Could you check a few things on this model? Use its own coordinates, in mm. Face numbers are marked on the shaded views. A direction names the side the tool comes from. Give positions to 0.01 mm unless a question says otherwise; leave off trailing zeros.
1. For the marked faces 1, 2 and 3, which set-ups out of +Z, -Z, +X, -X, +Y, -Y let a thin tool reach every point of the face, with its end or its side?
2. I need wall thicknesses on line 1 along X through (y, z) = (43, -130); line 2 along Y through (x, z) = (172, 88); line 3 along X through (y, z) = (-480, 148.5). Which ranges of each line are inside material? Lowest first, please.
3. Imagine slicing it at B-B (y = -230). Count the separate pieces of the cut face and the enclosed holes in it, plus the area to 3 significant figures.
4. Thinking about a two-plate mould opening in Y: for the marked faces 4, 5, 6 and 7, which applies, +Y half, -Y half, draft (parallel to the pull), parting line (faces both ways), or undercut?
5. For P1, Ø1.5, axis at x = 112.5, y = -453.5, coming from the +Z side; P2, Ø4, axis at x = 325, z = -55, coming from the +Y side; P3, Ø12, axis at y = -140, z = 74.5, coming from the +X side, each with a flat end and sliding along its axis, tell me the tip position at first contact or that it passes through.
```python
from build123d import *

# Parameters (mm, degrees)
SKETCH2_R           = 30
SKETCH2_R_2         = 105
SKETCH2_R_3         = 28.090856429
SKETCH2_R_4         = 15
BOSS_EXTRUDE2_DEPTH = 50
SKETCH5_R           = 30
CUT_EXTRUDE1_DEPTH  = 10
CHAMFER2_SIZE       = 10
BOSS_EXTRUDE3_START = 100
SKETCH6_R           = 145
SKETCH6_R_2         = 105
BOSS_EXTRUDE3_DEPTH = 100
CUT_EXTRUDE2_START  = -10
SKETCH9_R           = 30
SKETCH9_R_2         = 15
CUT_EXTRUDE2_DEPTH  = 10
SWEEP3_OUTLINE_R    = 145
SWEEP3_OUTLINE_R_2  = 105
SWEEP3_ANGLE        = 90
SKETCH12_R          = 145
SKETCH12_R_2        = 105
BOSS_EXTRUDE5_DEPTH = 100
BOSS_EXTRUDE6_DEPTH = 50
SKETCH14_R          = 105
CUT_EXTRUDE5_DEPTH  = 50
SKETCH17_R          = 30
SKETCH17_R_2        = 15
CUT_EXTRUDE6_DEPTH  = 10
SKETCH18_R          = 15
CUT_EXTRUDE7_DEPTH  = 100
CHAMFER3_SIZE       = 10


# Read off the part's stored shape, not the designer's step: Sweep3
with BuildPart() as part:
    # Sketch2 → Boss-Extrude2 (new body)
    # profile 1 of 5: a face of its own
    with BuildSketch(Plane(origin=(0, 0, 0), x_dir=(1, 0, 0), z_dir=(0, 1, 0))):
        with BuildLine():
            Line((-180, -130), (-180, -160))
            ThreePointArc((-180, -160), (-174.142135624, -174.142135624), (-160, -180))
            Line((-160, -180), (160, -180))
            ThreePointArc((160, -180), (174.142135624, -174.142135624), (180, -160))
            Line((180, -160), (180, 160))
            ThreePointArc((180, 160), (174.142135624, 174.142135624), (160, 180))
            Line((160, 180), (-160, 180))
            ThreePointArc((-160, 180), (-174.142135624, 174.142135624), (-180, 160))
            Line((-180, 160), (-180, -130))
        make_face()
        with Locations((-130, -130)):
            Circle(SKETCH2_R, mode=Mode.SUBTRACT)
        with Locations((130, -130)):
            Circle(SKETCH2_R, mode=Mode.SUBTRACT)
        with Locations((-130, 130)):
            Circle(SKETCH2_R, mode=Mode.SUBTRACT)
        with Locations(Location((0, 0, 0), (0, 0, 270))):
            Circle(SKETCH2_R_2, mode=Mode.SUBTRACT)
        with Locations((130, 130)):
            Circle(SKETCH2_R_3, mode=Mode.SUBTRACT)
    # profile 2 of 5: a face of its own
    with BuildSketch(Plane(origin=(0, 0, 0), x_dir=(1, 0, 0), z_dir=(0, 1, 0))):
        with Locations((-130, 130)):
            Circle(SKETCH2_R)
        with Locations(Location((-130, 130, 0), (0, 0, 270))):
            Circle(SKETCH2_R_4, mode=Mode.SUBTRACT)
    # profile 3 of 5: a face of its own
    with BuildSketch(Plane(origin=(0, 0, 0), x_dir=(1, 0, 0), z_dir=(0, 1, 0))):
        with Locations((130, 130)):
            Circle(SKETCH2_R_3)
        with Locations(Location((130, 130, 0), (0, 0, 270))):
            Circle(SKETCH2_R_4, mode=Mode.SUBTRACT)
    # profile 4 of 5: a face of its own
    with BuildSketch(Plane(origin=(0, 0, 0), x_dir=(1, 0, 0), z_dir=(0, 1, 0))):
        with Locations((-130, -130)):
            Circle(SKETCH2_R)
        with Locations(Location((-130, -130, 0), (0, 0, 270))):
            Circle(SKETCH2_R_4, mode=Mode.SUBTRACT)
    # profile 5 of 5: a face of its own
    with BuildSketch(Plane(origin=(0, 0, 0), x_dir=(1, 0, 0), z_dir=(0, 1, 0))):
        with Locations((130, -130)):
            Circle(SKETCH2_R)
        with Locations(Location((130, -130, 0), (0, 0, 270))):
            Circle(SKETCH2_R_4, mode=Mode.SUBTRACT)
    extrude(amount=BOSS_EXTRUDE2_DEPTH)

    # Sketch5 → Cut-Extrude1 (cut)
    with BuildSketch(Plane(origin=(0, 50, 0), x_dir=(1, 0, 0), z_dir=(0, 1, 0))):
        with Locations(Location((-130, 130, 0), (0, 0, 270))):
            Circle(SKETCH5_R)
        with Locations(Location((130, 130, 0), (0, 0, 270))):
            Circle(SKETCH5_R)
        with Locations(Location((-130, -130, 0), (0, 0, 270))):
            Circle(SKETCH5_R)
    extrude(amount=-CUT_EXTRUDE1_DEPTH, mode=Mode.SUBTRACT)

    # Chamfer2
    chamfer2_edges = [part.edges().sort_by_distance(p)[0] for p in [
        (0, 50, -105),
    ]]
    chamfer(chamfer2_edges, length=CHAMFER2_SIZE)

    # Sketch6 → Boss-Extrude3 (add)
    with BuildSketch(Plane.XZ.offset(BOSS_EXTRUDE3_START)):
        with Locations(Location((0, 0, 0), (0, 0, 90))):
            Circle(SKETCH6_R)
        with Locations(Location((0, 0, 0), (0, 0, 270))):
            Circle(SKETCH6_R_2, mode=Mode.SUBTRACT)
    extrude(amount=-BOSS_EXTRUDE3_DEPTH)

    # Sketch9 → Cut-Extrude2 (cut)
    with BuildSketch(Plane(origin=(0, 50, 0), x_dir=(1, 0, 0), z_dir=(0, 1, 0)).offset(CUT_EXTRUDE2_START)):
        with Locations(Location((130, -130, 0), (0, 0, 270))):
            Circle(SKETCH9_R)
        with Locations(Location((130, -130, 0), (0, 0, 270))):
            Circle(SKETCH9_R_2, mode=Mode.SUBTRACT)
    extrude(amount=CUT_EXTRUDE2_DEPTH, mode=Mode.SUBTRACT)

    # Sweep3 outline → Sweep3 (revolve)
    with BuildSketch(Plane(origin=(260, -100, 0), x_dir=(-1, 0, 0), z_dir=(0, 1, 0))):
        with Locations((260, 0)):
            Circle(SWEEP3_OUTLINE_R)
        with Locations((260, 0)):
            Circle(SWEEP3_OUTLINE_R_2, mode=Mode.SUBTRACT)
    revolve(axis=Axis((260, -100, 0), (0, 0, 1)), revolution_arc=SWEEP3_ANGLE)

    # Sketch12 → Boss-Extrude5 (add)
    with BuildSketch(Plane(origin=(260, 0, 0), x_dir=(0, 0, -1), z_dir=(1, 0, 0))):
        with Locations(Location((0, -360, 0), (0, 0, 270))):
            Circle(SKETCH12_R)
        with Locations(Location((0, -360, 0), (0, 0, 270))):
            Circle(SKETCH12_R_2, mode=Mode.SUBTRACT)
    extrude(amount=BOSS_EXTRUDE5_DEPTH)

    # Sketch13 → Boss-Extrude6 (add)
    with BuildSketch(Plane(origin=(360, 0, 0), x_dir=(0, 0, -1), z_dir=(1, 0, 0))):
        with BuildLine():
            Line((-170, -540), (170, -540))
            ThreePointArc((170, -540), (177.071067812, -537.071067812), (180, -530))
            Line((180, -530), (180, -190))
            ThreePointArc((180, -190), (177.071067812, -182.928932188), (170, -180))
            Line((170, -180), (-170, -180))
            ThreePointArc((-170, -180), (-177.071067812, -182.928932188), (-180, -190))
            Line((-180, -190), (-180, -530))
            ThreePointArc((-180, -530), (-177.071067812, -537.071067812), (-170, -540))
        make_face()
    extrude(amount=BOSS_EXTRUDE6_DEPTH)

    # Sketch14 → Cut-Extrude5 (cut)
    with BuildSketch(Plane(origin=(410, 0, 0), x_dir=(0, 0, -1), z_dir=(1, 0, 0))):
        with Locations(Location((0, -369.029004143, 0), (0, 0, 90))):
            Circle(SKETCH14_R)
    extrude(amount=-CUT_EXTRUDE5_DEPTH, mode=Mode.SUBTRACT)

    # Sketch17 → Cut-Extrude6 (cut)
    # profile 1 of 4: a face of its own
    with BuildSketch(Plane(origin=(410, 0, 0), x_dir=(0, 0, -1), z_dir=(1, 0, 0))):
        with Locations(Location((-130, -230, 0), (0, 0, 90))):
            Circle(SKETCH17_R)
        with Locations(Location((-130, -230, 0), (0, 0, 90))):
            Circle(SKETCH17_R_2, mode=Mode.SUBTRACT)
    # profile 2 of 4: a face of its own
    with BuildSketch(Plane(origin=(410, 0, 0), x_dir=(0, 0, -1), z_dir=(1, 0, 0))):
        with Locations(Location((-130, -490, 0), (0, 0, 90))):
            Circle(SKETCH17_R)
        with Locations(Location((-130, -490, 0), (0, 0, 90))):
            Circle(SKETCH17_R_2, mode=Mode.SUBTRACT)
    # profile 3 of 4: a face of its own
    with BuildSketch(Plane(origin=(410, 0, 0), x_dir=(0, 0, -1), z_dir=(1, 0, 0))):
        with Locations(Location((130, -490, 0), (0, 0, 90))):
            Circle(SKETCH17_R)
        with Locations(Location((130, -490, 0), (0, 0, 90))):
            Circle(SKETCH17_R_2, mode=Mode.SUBTRACT)
    # profile 4 of 4: a face of its own
    with BuildSketch(Plane(origin=(410, 0, 0), x_dir=(0, 0, -1), z_dir=(1, 0, 0))):
        with Locations(Location((130, -230, 0), (0, 0, 90))):
            Circle(SKETCH17_R)
        with Locations(Location((130, -230, 0), (0, 0, 90))):
            Circle(SKETCH17_R_2, mode=Mode.SUBTRACT)
    extrude(amount=-CUT_EXTRUDE6_DEPTH, mode=Mode.SUBTRACT)

    # Sketch18 → Cut-Extrude7 (cut)
    with BuildSketch(Plane(origin=(410, 0, 0), x_dir=(0, 0, -1), z_dir=(1, 0, 0))):
        with Locations(Location((-130, -230, 0), (0, 0, 90))):
            Circle(SKETCH18_R)
        with Locations(Location((130, -230, 0), (0, 0, 90))):
            Circle(SKETCH18_R)
        with Locations(Location((-130, -490, 0), (0, 0, 90))):
            Circle(SKETCH18_R)
        with Locations(Location((130, -490, 0), (0, 0, 90))):
            Circle(SKETCH18_R)
    extrude(amount=-CUT_EXTRUDE7_DEPTH, mode=Mode.SUBTRACT)

    # Chamfer3
    chamfer3_edges = [part.edges().sort_by_distance(p)[0] for p in [
        (410, -474.029004143, 0),
    ]]
    chamfer(chamfer3_edges, length=CHAMFER3_SIZE)


solid = part.part
```
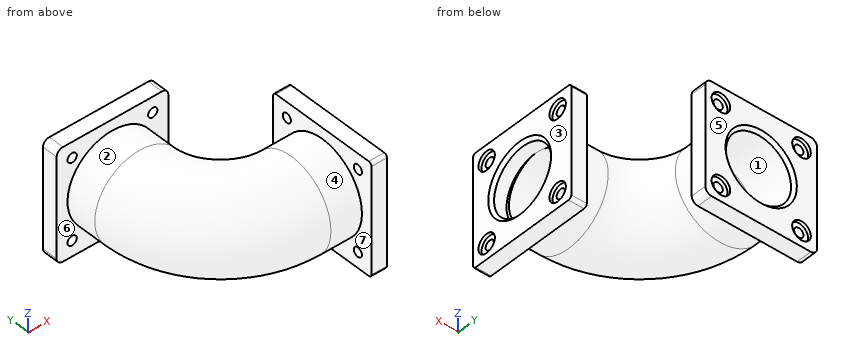
Derived:
1. face 1: +Y
1. face 2: none
1. face 3: +Z, -Z, +X, +Y, -Y
2. line 1: x = -180 to -160, -100 to 100, 160 to 180
2. line 2: y = -464.78 to -404.83, -282.62 to -214.94, 0 to 50
2. line 3: x = 360 to 400
3. separate pieces: 3
3. enclosed holes: 1
3. area: 71,600 mm2
4. face 4: parting line
4. face 5: +Y half
4. face 6: undercut
4. face 7: draft
5. P1: stops at z = 77.91
5. P2: stops at y = -225.03
5. P3: stops at x = 134.53
